from build123d import *

# Parameters (mm, degrees)
SKETCH001_W  = 145.57
SKETCH001_H  = 76.477117
PAD_DEPTH    = 3
PAD001_DEPTH = 151
SKETCH004_W  = 234.832214
SKETCH004_H  = 173.073643
POCKET_DEPTH = 200
PAD002_DEPTH = 3
SKETCH003_R  = 1.4
PAD003_DEPTH = 10


with BuildPart() as part:
    # Sketch001 → Pad (new body)
    with BuildSketch(Plane.XY):
        with Locations((0, -3.210938)):
            Rectangle(SKETCH001_W, SKETCH001_H)
    extrude(amount=-PAD_DEPTH)

    # Sketch → Pad001 (join)
    with BuildSketch(Plane.XY):
        Polygon((51.785, -26.449496), (57.785, -26.449496), (57.785, 20.027621), (-57.785, 20.027621), (-57.785, -26.449496), (-51.785, -26.449496), (-51.785, 14.027621), (51.785, 14.027621), align=None)
    extrude(amount=PAD001_DEPTH)

    # Sketch004 (on DatumPlane) → Pocket (cut)
    with BuildSketch(Plane(origin=(0, -37.819078, 1.02606), x_dir=(1, 0, 0), z_dir=(0, -0.939693, 0.34202))):
        with Locations((5.697174, 86.536822)):
            Rectangle(SKETCH004_W, SKETCH004_H)
    extrude(amount=POCKET_DEPTH, mode=Mode.SUBTRACT)

    # Sketch002 (on DatumPlane) → Pad002 (join)
    with BuildSketch(Plane(origin=(0, -35, 0), x_dir=(1, 0, 0), z_dir=(0, -0.939693, 0.34202))):
        Polygon((-57.785, 160.89), (57.785, 160.89), (57.785, 25), (51.785, 25), (51.785, 47), (-5.215, 47), (-5.215, 25), (-57.785, 25), align=None)
    extrude(amount=PAD002_DEPTH)

    # Sketch003 (on DatumPlane) → Pad003 (join)
    with BuildSketch(Plane(origin=(0, -35, 0), x_dir=(1, 0, 0), z_dir=(0, -0.939693, 0.34202))):
        with Locations((-54.61, 157.715)):
            Circle(SKETCH003_R)
        with Locations((54.61, 157.715)):
            Circle(SKETCH003_R)
        with Locations((54.61, 28.175)):
            Circle(SKETCH003_R)
        with Locations((-54.61, 28.175)):
            Circle(SKETCH003_R)
    extrude(amount=PAD003_DEPTH)


solid = part.part
Could you check a few things on this model? Use its own coordinates, in mm. A direction names the side the tool comes from. Give positions to 0.01 mm unless a question says otherwise; leave off trailing zeros. Order: outer loops, then holes, each group sorted by start corner. A loop starts at its lowest first (then second) coordinate and runs counter-clockwise, first axis right, second up.
Item 1: If we section it at D-D, the plane z = 18.5: Write out the boundary of the cut face in (x, y) (1 decimal), plus the area to 3 significant figures.
Item 2: If we section it at B-B, the plane z = 113: Write out the boundary of the cut face in (x, y) (3 decimals).
Item 3: I'm going to push flat-ended pins straight in: pin 1 (3 mm diameter, centred on y = -22, z = 34, fed in from +X) (3 decimals); pin 2 (1.5 mm diameter, centred on x = 40, z = 42.5, fed in from +Y); pin 3 (15 mm diameter, centred on y = 1.5, z = 86.5, fed in from -X) (3 decimals). Where does each tip first touch, or does it pass through?
Item 4: If we section it at C-C, the plane y = -16.5: Write out the boundary of the cut face in (x, z) (3 decimals), plus the area to 3 significant figures.
Item 5: For faces 4 (the face through (-51.785, -2, 51)), 5 (the face through (55, -26.449, 12)), 6 (the face through (-57.785, -2, 55)), 7 (the face through (1, 20.028, 74)), 8 (the face through (-5.215, -24, 34)), which set-ups out of +Z, -Z, +X, -X, +Y, -Y let a thin tool reach every point of the face, with its end or its side?
Item 6: If we mould it in two halves opening along Z, with no side actions, what happens to faces 1 (the face through (57.785, -1, 57)), 2 (the face through (-1, -3, -3)), 3 (the face through (51.785, -3, 51))? For each: pulls with the +Z half, pulls with the -Z half, needs draft (parallel to the pull), parting line crosses it, or undercut.
Item 7: If we section it at A-A, the plane x = 32: Write out the boundary of the cut face in (y, z), plus the area to 3 significant figures.
Item 8: I need wall thicknesses on line 1 (X direction, y = 6, z = 34) (3 decimals); line 2 (Z direction, x = -60, y = 8); line 3 (Y direction, x = 4.5, z = 37.5). Which ranges of each line are inside material? Lowest first, please.
Values:
1. outline: (-57.8, -26.4) - (-51.8, -26.4) - (-51.8, 14) - (51.8, 14) - (51.8, -26.4) - (57.8, -26.4) - (57.8, 20) - (-57.8, 20) - close
1. area: 1,180 mm2
2. outline: (-57.785, 2.936) - (57.785, 2.936) - (57.785, 20.028) - (-57.785, 20.028) - close; hole (-51.785, 6.129) - (51.785, 6.129) - (51.785, 14.028) - (-51.785, 14.028) - close
3. pin 1: stops at x = 57.785
3. pin 2: stops at y = 20.03
3. pin 3: stops at x = -57.785
4. outline: (-72.785, -3) - (72.785, -3) - (72.785, 0) - (57.785, 0) - (57.785, 59.6) - (-57.785, 59.6) - (-57.785, 0) - (-72.785, 0) - close; hole (-51.785, 0) - (51.785, 0) - (51.785, 50.828) - (-51.785, 50.828) - close
4. area: 2,060 mm2
5. face 4: none
5. face 5: +X, -X, -Y
5. face 6: +Z, -X, +Y, -Y
5. face 7: +Z, +X, -X, +Y
5. face 8: -Y
6. face 1: needs draft
6. face 2: pulls with the -Z half
6. face 3: undercut
7. outline: (-41.45, -3) - (35.03, -3) - (35.03, 0) - (20.03, 0) - (20.03, 151) - (19.96, 151) - (20.03, 151.19) - (17.21, 152.21) - (-21.74, 45.19) - (-18.93, 44.17) - (14.03, 134.7) - (14.03, 0) - (-41.45, 0) - close
7. area: 1,430 mm2
8. line 1: x = -57.785 to -51.785, 51.785 to 57.785
8. line 2: z = -3 to 0
8. line 3: y = 14.03 to 20.03
